```python
from build123d import *

# Parameters (mm, degrees)
SKETCH1_W           = 90
SKETCH1_H           = 90
BOSS_EXTRUDE1_DEPTH = 37
FILLET1_R           = 5
SKETCH2_R           = 18
BOSS_EXTRUDE2_DEPTH = 5
SKETCH3_R           = 6
BOSS_EXTRUDE3_DEPTH = 27
BOSS_EXTRUDE5_DEPTH = 105
CHAMFER1_SIZE       = 0.5
SKETCH5_R           = 3.25
CUT_EXTRUDE1_DEPTH  = 44.5


with BuildPart() as part:
    # Sketch1 → Boss-Extrude1 (new body)
    with BuildSketch(Plane.XY):
        Rectangle(SKETCH1_W, SKETCH1_H)
    extrude(amount=BOSS_EXTRUDE1_DEPTH)

    # Fillet1
    fillet1_edges = [part.edges().sort_by_distance(p)[0] for p in [
        (45, -45, 18.5),
        (-45, -45, 18.5),
        (-45, 45, 18.5),
        (45, 45, 18.5),
    ]]
    fillet(fillet1_edges, radius=FILLET1_R)

    # Sketch2 → Boss-Extrude2 (add)
    with BuildSketch(Plane.XY.offset(37)):
        with Locations((0, 18)):
            Circle(SKETCH2_R)
    extrude(amount=BOSS_EXTRUDE2_DEPTH)

    # Sketch3 → Boss-Extrude3 (add)
    with BuildSketch(Plane.XY.offset(42)):
        with Locations((0, 18)):
            Circle(SKETCH3_R)
    extrude(amount=BOSS_EXTRUDE3_DEPTH)

    # Sketch4 → Boss-Extrude5 (add)
    with BuildSketch(Plane(origin=(0, 0, 0), x_dir=(-1, 0, 0), z_dir=(0, 0, -1))):
        with BuildLine():
            Line((-30, 45), (30, 45))
            ThreePointArc((30, 45), (40.606601718, 40.606601718), (45, 30))
            Line((45, 30), (45, -30))
            ThreePointArc((45, -30), (40.606601718, -40.606601718), (30, -45))
            Line((30, -45), (-30, -45))
            ThreePointArc((-30, -45), (-40.606601718, -40.606601718), (-45, -30))
            Line((-45, -30), (-45, 30))
            ThreePointArc((-45, 30), (-40.606601718, 40.606601718), (-30, 45))
        make_face()
    extrude(amount=BOSS_EXTRUDE5_DEPTH)

    # Chamfer1
    chamfer1_edges = [part.edges().sort_by_distance(p)[0] for p in [
        (-6, 18, 69),
    ]]
    chamfer(chamfer1_edges, length=CHAMFER1_SIZE)

    # Sketch5 → Cut-Extrude1 (cut)
    with BuildSketch(Plane.XY.offset(37)):
        with Locations((-36.8, 36.8)):
            Circle(SKETCH5_R)
        with Locations((36.8, 36.8)):
            Circle(SKETCH5_R)
        with Locations((36.8, -36.8)):
            Circle(SKETCH5_R)
        with Locations((-36.8, -36.8)):
            Circle(SKETCH5_R)
    extrude(amount=-CUT_EXTRUDE1_DEPTH, mode=Mode.SUBTRACT)


solid = part.part
```
Could you check a few things on this model? Use its own coordinates, in mm. A direction names the side the tool comes from. Round coordinates to 2 decimals unless told otherwise and drop trailing zeros. Order: outer loops, then holes, each group sorted by start corner. A loop starts at its lowest first (then second) coordinate and runs counter-clockwise, first axis right, second up. Notation, with made-up numbers: (-34, -10) -> (6, -10) arc R19 ccw to (6, 4) -> close; hole circle Ø11 at (43.5, 49.25). An arc over 180 degrees is marked (long way). One line per question, with ' | ' between items.
Q1. We'd pull the mould along X, two halves only. Please class faces 1 (the face through (-37.223, 40.022, 15.061)), 2 (the face through (-1, 45, -35)), 3 (the face through (-40.49, 40.72, -51.76)): released by +X, released by -X, zero draft, split by the parting line, or undercut.
Computed values:
face 1: undercut | face 2: zero draft | face 3: released by -X
Q2. If we section it at B-B on y = 18: Write out the boundary of the cut face in (x, z).
Computed values:
outline: (-45, -105) -> (45, -105) -> (45, 37) -> (18, 37) -> (18, 42) -> (6, 42) -> (6, 68.5) -> (5.5, 69) -> (-5.5, 69) -> (-6, 68.5) -> (-6, 42) -> (-18, 42) -> (-18, 37) -> (-45, 37) -> close
Q3. If I drill on line 1 (Y direction, x = -36.8, z = 13); line 2 (Y direction, x = 35.5, z = 34.5); line 3 (X direction, y = 36, z = 21), over which ranges is the centre line in solid material (lowest first)? Write a range as from..to.
Computed values:
line 1: -45..-40.05, -33.55..33.55, 40.05..45 | line 2: -45..-39.78, -33.82..33.82, 39.78..45 | line 3: -45..-39.95, -33.65..33.65, 39.95..45
Q4. Which directions (+Z, -Z, +X, -X, +Y, -Y) give clear straight access to the entire face, cutting with the end or side of a thin tool? Please do faces 4 (the face through (-41, -41, 0)), 5 (the face through (-3.902, 0.428, 39.465)), 6 (the face through (41, -41, 0)).
Computed values:
face 4: -Z, -X, -Y | face 5: +Z | face 6: -Z, +X, -Y
Q5. If we section it at C-C on x = 0: Write out the boundary of the cut face in (y, z), plus the area to 3 significant figures.
Computed values:
outline: (-45, -105) -> (45, -105) -> (45, 37) -> (36, 37) -> (36, 42) -> (24, 42) -> (24, 68.5) -> (23.5, 69) -> (12.5, 69) -> (12, 68.5) -> (12, 42) -> (0, 42) -> (0, 37) -> (-45, 37) -> close | area: 13,300 mm²
Q6. I'm going to push flat-ended pins straight in: pin 1 (3 mm diameter, centred on x = -36.5, y = 37.5, fed in from +Z); pin 2 (5 mm diameter, centred on x = 37, y = 35.5, fed in from +Z); pin 3 (10 mm diameter, centred on x = 10.5, y = 35, fed in from +Z). Where does each tip first touch, or does it pass through?
Computed values:
pin 1: z = -7.5 | pin 2: z = 37 | pin 3: z = 42
Q7. If we section it at D-D on z = -31.5: Write out the boundary of the cut face in (x, y), plus the area to 3 significant figures.
Computed values:
outline: (-45, -30) arc R15 ccw to (-30, -45) -> (30, -45) arc R15 ccw to (45, -30) -> (45, 30) arc R15 ccw to (30, 45) -> (-30, 45) arc R15 ccw to (-45, 30) -> close | area: 7,910 mm²
Q8. If we section it at A-A on z = -3.5: Write out the boundary of the cut face in (x, y).
Computed values:
outline: (-45, -30) arc R15 ccw to (-30, -45) -> (30, -45) arc R15 ccw to (45, -30) -> (45, 30) arc R15 ccw to (30, 45) -> (-30, 45) arc R15 ccw to (-45, 30) -> close; hole circle Ø6.5 at (-36.8, -36.8); hole circle Ø6.5 at (-36.8, 36.8); hole circle Ø6.5 at (36.8, -36.8); hole circle Ø6.5 at (36.8, 36.8)
